from build123d import *

# Parameters (mm, degrees)
F1_DEPTH = 19.05
F2_R     = 5.08
F3_R     = 2.2225
F4_DEPTH = 12.0466452


# Not quite as in the source:
# - ends of sketch curves that miss each other by under 0.0002 mm in the source are joined


with BuildPart() as f1:
    # F0 (on Front) → F1 (new body)
    with BuildSketch(Plane.XZ):
        with BuildLine():
            Line((-12.0627648, -8.5602826), (-12.0627648, -12.0865646))
            Line((-12.0627648, -12.0865646), (-5.1851306, -12.0865646))
            ThreePointArc((-5.1851306, -12.0865646), (1.4407652276, -13.3594055352), (7.5600808337, -16.2013401088))
            Line((7.5600808337, -16.2013401088), (8.6856062, -16.8927272))
            ThreePointArc((8.6856062, -16.8927272), (8.9620015383, -17.2612655931), (8.8635755348, -17.7112866346))
            Line((8.8635755348, -17.7112866346), (7.5629516, -19.149187))
            Line((7.5629516, -19.149187), (10.5785158, -19.149187))
            ThreePointArc((10.5785158, -19.149187), (11.6521464417, -18.2940868169), (12.0627642118, -16.9843959643))
            Line((12.0627642118, -16.9843959643), (12.0627394, -13.1420616))
            Line((12.0627394, -13.1420616), (8.6250272, -10.822813))
            Line((8.6250272, -10.822813), (8.6250272, 19.149187))
            Line((8.6250272, 19.149187), (-1.0269728, 19.149187))
            Line((-1.0269728, 19.149187), (-1.0269728, -7.1035418))
            Line((-1.0269728, -7.1035418), (-10.6173016, -7.1035418))
            ThreePointArc((-10.6173016, -7.1035418), (-11.6378820464, -7.5363696119), (-12.0627648, -8.5602826))
        make_face()
    extrude(amount=F1_DEPTH)

    # F2
    f2_edges = [f1.edges().sort_by_distance(p)[0] for p in [
        (3.799027, -19.05, 19.149187),
        (3.799027, 0, 19.149187),
    ]]
    fillet(f2_edges, radius=F2_R)

    # F3 (on face) → F4 (cut, through all)
    with BuildSketch(Plane.XY.offset(-7.1035418)):
        with Locations((-6.7287706383, -9.525)):
            Circle(F3_R)
    extrude(amount=-F4_DEPTH, mode=Mode.SUBTRACT)


solid = f1.part
Model file for the job. Use its own axes, mm. A direction names the side the tool comes from. Give positions to 0.01 mm unless a question says otherwise; leave off trailing zeros. Order: outer loops, then holes, each group sorted by start corner. A loop starts at its lowest first (then second) coordinate and runs counter-clockwise, first axis right, second up. Notation, with made-up numbers: M 72,43 L 81,43 A13 ccw 81,61 Z; hole C -29,9 d7. An arc over 180 degrees is marked long. Write item = value, one per line.
Q1. Drill centre lines: line 1 (Z direction, x = -9.5, y = -14.75); line 2 (X direction, y = -3.5, z = 9); line 3 (Y direction, x = -7.25, z = -12). Where is each one in solid material? Low to high. Write a range as [from, to].
Derived:
line_1 = [-12.09, -7.1]
line_2 = [-1.03, 8.63]
line_3 = [-19.05, -11.69], [-7.36, 0]
Q2. Two-plate mould, pull along Z, no slides. Class faces 1 (the cylindrical face through (-7.211, -11.695, -9.587)), 2 (the flat face through (-9.4, -9.4, -12.087)), 3 (the flat face through (8.11, -9.39, -16.54)), 4 (the cylindrical face through (8.96, -9.39, -17.25)): pulls with the +Z half, pulls with the -Z half, needs draft (parallel to the pull), parting line crosses it, or undercut.
Derived:
face_1 = needs draft
face_2 = pulls with the -Z half
face_3 = undercut
face_4 = undercut
Q3. Flat gauge pins, fed straight in: pin 1 (6 mm diameter, centred on x = -8.5, y = -16.5, fed in from -Z); pin 2 (5 mm diameter, centred on x = -6.73, y = -9.52, fed in from -Z); pin 3 (9.5 mm diameter, centred on y = -5.5, z = 6.5, fed in from -X). Where does each tip first touch, or does it go through?
Derived:
pin_1 = -12.09
pin_2 = -12.17
pin_3 = -1.03
Q4. Cut at B-B, the plane z = 0.5. List the corners of the cut face in (x, y), then the cut area to 3 significant figures.
Derived:
outline = M -1.03,-19.05 L 8.63,-19.05 L 8.63,0 L -1.03,0 Z
area = 184 mm2
Q5. Cut at C-C, the plane x = 3. List the corners of the cut face in (y, z).
Derived:
outline = M -19.05,-13.91 L 0,-13.91 L 0,14.07 A5.08 ccw -5.08,19.15 L -13.97,19.15 A5.08 ccw -19.05,14.07 Z
Q6. Tool access for faces 5 (the flat face through (-6, -7, -7.104)), 6 (the flat face through (8.625, -9, 4)), 7 (the flat face through (8.22, -9.39, -18.42)): list every direction of +Z, -Z, +X, -X, +Y, -Y with a clear straight run to the whole face (end or side of a thin tool).
Derived:
face_5 = +Z, -X, +Y, -Y
face_6 = +Z, +X, +Y, -Y
face_7 = -X, +Y, -Y
Q7. Cut at A-A, the plane y = -12.5. List the corners of the cut face in (x, z).
Derived:
outline = M -12.06,-12.09 L -5.19,-12.09 A27.61 cw 7.56,-16.2 L 8.69,-16.89 A0.55 cw 8.86,-17.71 L 7.56,-19.15 L 10.58,-19.15 A2.34 ccw 12.06,-16.98 L 12.06,-13.14 L 8.63,-10.82 L 8.63,19.15 L -1.03,19.15 L -1.03,-7.1 L -10.62,-7.1 A1.46 ccw -12.06,-8.56 Z
